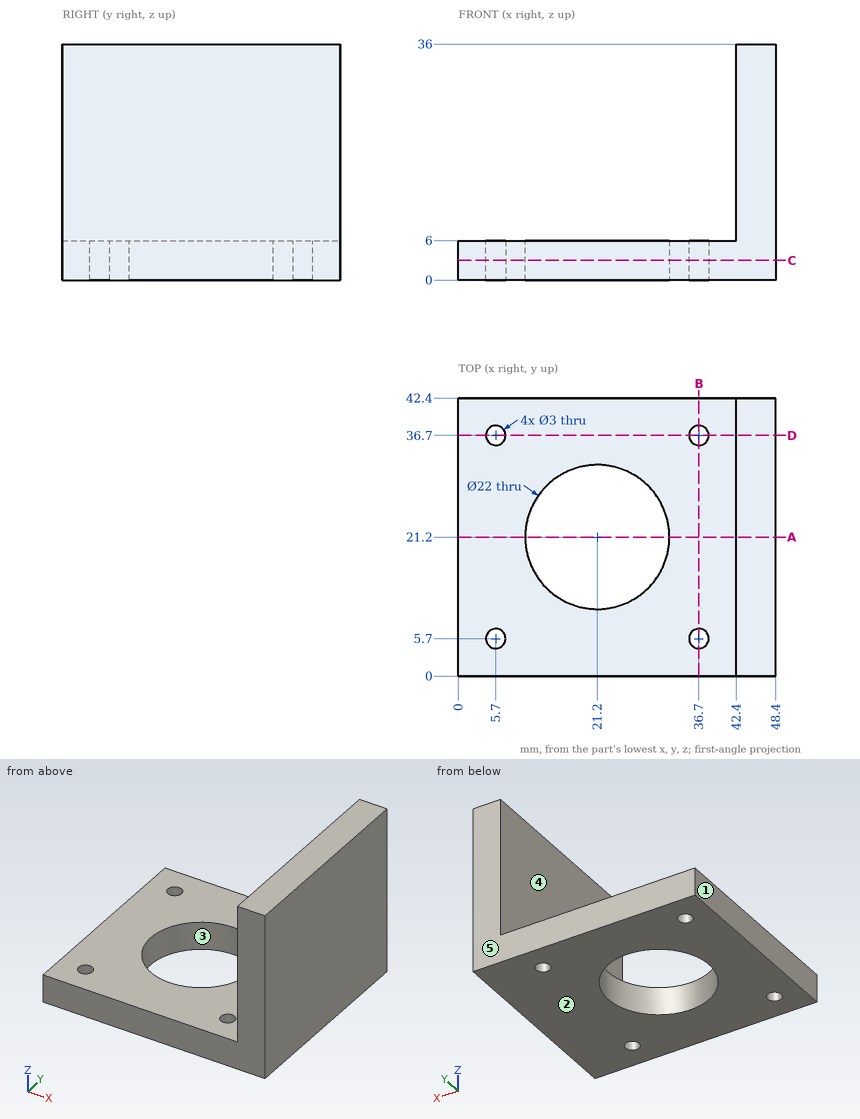
The drawing under review shows one solid part. Ordinate dimensions are in mm from its lowest x, y, z. A direction names the side the tool comes from. Round coordinates to 2 decimals unless told otherwise and drop trailing zeros. Order: outer loops, then holes, each group sorted by start corner. A loop starts at its lowest first (then second) coordinate and runs counter-clockwise, first axis right, second up. Notation, with made-up numbers: (9, 57.25) -> (34, 57.25) arc R12 ccw to (34, 71.25) -> close; hole circle Ø6 at (-24, 66). An arc over 180 degrees is marked (long way). Return JSON: item names as keys, results as strings.
1. The part is to be moulded in two halves that separate along X. For the marked faces 1, 2 and 3, say which applies: +X half, -X half, draft (parallel to the pull), parting line (faces both ways), or undercut.
Answer block:
{"face 1": "-X half", "face 2": "draft", "face 3": "undercut"}
2. Take a section at A-A (y = 21.2). Write out the cut boundary in (x, z), then the cut area to 3 significant figures.
Answer block:
{"outline": "(0, 0) -> (10.2, 0) -> (10.2, 6) -> (0, 6) -> close; (32.2, 0) -> (48.4, 0) -> (48.4, 36) -> (42.4, 36) -> (42.4, 6) -> (32.2, 6) -> close", "area": "338 mm²"}
3. Take a section at B-B (x = 36.7). Write out the cut boundary in (y, z).
Answer block:
{"outline": "(0, 0) -> (4.2, 0) -> (4.2, 6) -> (0, 6) -> close; (7.2, 0) -> (35.2, 0) -> (35.2, 6) -> (7.2, 6) -> close; (38.2, 0) -> (42.4, 0) -> (42.4, 6) -> (38.2, 6) -> close"}
4. Insertion check: P1, Ø3, axis at y = 28.5, z = 26.5, coming from the -X side; P2, Ø3, axis at x = 29.5, y = 10, coming from the +Z side; P3, Ø2.5, axis at x = 36.7, y = 36.7, coming from the +Z side. Each pin has a flat end and moves straight along its axis. Give the tip position at first contact, or say it passes through.
Answer block:
{"P1": "stops at x = 42.4", "P2": "stops at z = 6", "P3": "passes through"}
5. Take a section at C-C (z = 3). Write out the cut boundary in (x, y), then the cut area to 3 significant figures.
Answer block:
{"outline": "(0, 0) -> (48.4, 0) -> (48.4, 42.4) -> (0, 42.4) -> close; hole circle Ø3 at (5.7, 5.7); hole circle Ø3 at (5.7, 36.7); hole circle Ø22 at (21.2, 21.2); hole circle Ø3 at (36.7, 5.7); hole circle Ø3 at (36.7, 36.7)", "area": "1,640 mm²"}
6. For L1, parallel to Y at x = 36.7, z = 4.4; L2, parallel to X at y = 21, z = 4; L3, parallel to Z at x = 35, y = 27, list the stretches that pass through material, from the lowest coordinate up. Write a range as [from, to].
Answer block:
{"L1": "y = [0, 4.2], [7.2, 35.2], [38.2, 42.4]", "L2": "x = [0, 10.2], [32.2, 48.4]", "L3": "z = [0, 6]"}
7. Take a section at D-D (y = 36.7). Write out the cut boundary in (x, z), then the cut area to 3 significant figures.
Answer block:
{"outline": "(0, 0) -> (4.2, 0) -> (4.2, 6) -> (0, 6) -> close; (7.2, 0) -> (35.2, 0) -> (35.2, 6) -> (7.2, 6) -> close; (38.2, 0) -> (48.4, 0) -> (48.4, 36) -> (42.4, 36) -> (42.4, 6) -> (38.2, 6) -> close", "area": "434 mm²"}
8. For the marked faces 4 and 5, list the 3-axis set-ups (+Z, -Z, +X, -X, +Y, -Y) from which the entire face can be reached by the end or side of a thin tool; tool diameter is ignored.
Answer block:
{"face 4": "+Z, -X, +Y, -Y", "face 5": "+Z, -Z, +X, -X, +Y"}
